Here's how the part is built. I have some questions about the finished solid (model axes, mm). Face numbers are marked on the shaded views. A direction names the side the tool comes from. Round coordinates to 2 decimals unless told otherwise and drop trailing zeros. Loops run counter-clockwise (first coordinate to the right, second up) from the corner with the lowest first, then second, coordinate; pieces in that order, holes last. Notation, with made-up numbers: (-0.75, -7.75) - (58.25, -7.75) arc R22 cw to (58.25, 13.25) - close; hole circle Ø10 at (25.5, 89.5). An arc over 180 degrees is marked (long way). Return JSON: item names as keys, results as strings. Group by question number.
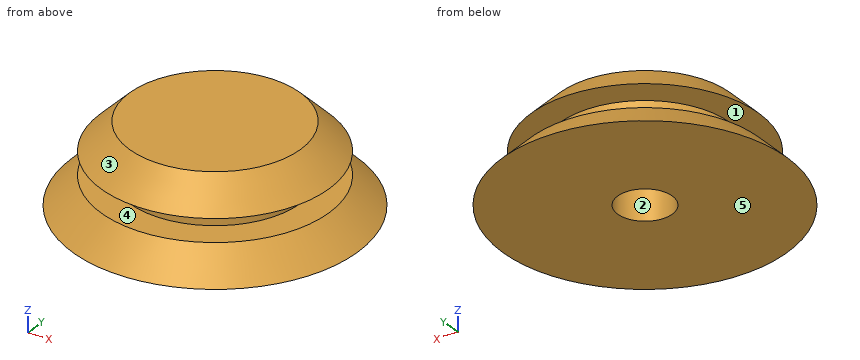
```python
from build123d import *


with BuildPart() as f1:
    # F0 (on Front) → F1 (revolve)
    with BuildSketch(Plane.XZ):
        Polygon((1.5875, 1.5875), (0, 0), (1.5875, 0), (1.5875, -1.27), (0, -1.27), (0, -2.8575), (2.69875, -2.8575), (4.826, -0.73025), (6.35, 0.79375), (6.35, 1.5875), align=None)
        Polygon((0, -2.8575), (0, -1.27), (-1.5875, -2.8575), align=None)
        Polygon((4.826, -2.8575), (4.826, -0.73025), (2.69875, -2.8575), align=None)
    revolve(axis=Axis((6.35, 0, 1.190625), (0, 0, -1)))


solid = f1.part
```
Q1. Imagine slicing it at A-A, the plane z = -2.45. List the corners of the cut face in (x, y) for me.
Q2. Please list where these lines run through material, in increasing order: line 1 (Z direction, x = 10, y = 3.5); line 2 (Y direction, x = 6.35, z = -2); line 3 (Z direction, x = 11.5, y = 2).
Q3. Will these pins go through, and if not, where does the flat tip stop? pin 1 Ø2 at (y, z) = (-5.5, -1.5) entering from +X; pin 2 Ø2 at (x, z) = (7, 0) entering from +Y; pin 3 Ø1 at (y, z) = (-2.5, -1.5) entering from -X.
Q4. If we mould it in two halves opening along X, with no side actions, what happens to the marked faces 1, 2 and 3? For each: +X half, -X half, draft (parallel to the pull), parting line (faces both ways), or undercut.
Q5. For the marked faces 4 and 5, which set-ups out of +Z, -Z, +X, -X, +Y, -Y let a thin tool reach every point of the face, with its end or its side?
Q6. Imagine slicing it at B-B, the plane z = -1.5. List the corners of the cut face in (x, y) for me.
Output values:
{
 "1": {"outline": "circle Ø15.06 at (6.35, 0); hole circle Ø3.05 at (6.35, 0)"},
 "2": {"line 1": "z = -2.86 to -1.27, 0 to 1.29", "line 2": "y = -7.08 to -1.52, 1.52 to 7.08", "line 3": "z = -2.86 to -1.27, 0 to 0.83"},
 "3": {"pin 1": "stops at x = 11.87", "pin 2": "stops at y = 6.35", "pin 3": "stops at x = -0.3"},
 "4": {"face 1": "draft", "face 2": "undercut", "face 3": "parting line"},
 "5": {"face 4": "none", "face 5": "-Z, +X, -X, +Y, -Y"},
 "6": {"outline": "circle Ø13.16 at (6.35, 0); hole circle Ø3.05 at (6.35, 0)"}
}
